The model under review builds one solid part; all positions refer to its coordinate system, in mm. A direction names the side the tool comes from. Round coordinates to 2 decimals unless told otherwise and drop trailing zeros. Loops run counter-clockwise (first coordinate to the right, second up) from the corner with the lowest first, then second, coordinate; pieces in that order, holes last. Notation, with made-up numbers: (67.5, -29.75) - (85.5, -29.75) arc R17 ccw to (85.5, -15.75) - close; hole circle Ø8 at (64, -31). An arc over 180 degrees is marked (long way). Answer as CSV lines item,"result".
from build123d import *

# Parameters (mm, degrees)
SKETCH1_W                                      = 104.000000026
SKETCH1_H                                      = 101.6
BOSS_EXTRUDE1_DEPTH                            = 10.16
SKETCH5_R                                      = 30.1625
BOSS_EXTRUDE2_DEPTH                            = 2.54
CBORE_FOR_6_SOCKET_HEAD_CAP_SCREW1_D           = 3.7973
CBORE_FOR_6_SOCKET_HEAD_CAP_SCREW1_CBORE_D     = 7.14502
CBORE_FOR_6_SOCKET_HEAD_CAP_SCREW1_CBORE_DEPTH = 3.5052
F_3_8_16_TAPPED_HOLE1_D                        = 7.9375
CBORE_FOR_M8_SBHCS1_D                          = 8.4
CBORE_FOR_M8_SBHCS1_CBORE_D                    = 14
CBORE_FOR_M8_SBHCS1_CBORE_DEPTH                = 4.4
CHAMFER1_SIZE                                  = 0.254
CHAMFER1_SIZE2                                 = 0.439940905
CHAMFER1_PART_2_SIZE                           = 0.254
CHAMFER1_PART_2_SIZE2                          = 0.439940905
CHAMFER2_SIZE                                  = 0.508


with BuildPart() as part:
    # Sketch1 → Boss-Extrude1 (new body)
    with BuildSketch(Plane(origin=(0, 0, 0), x_dir=(1, 0, 0), z_dir=(0, 1, 0))):
        with Locations((-52.000000013, 50.8)):
            Rectangle(SKETCH1_W, SKETCH1_H)
    extrude(amount=BOSS_EXTRUDE1_DEPTH)

    # Sketch5 → Boss-Extrude2 (add)
    with BuildSketch(Plane(origin=(0, 10.16, 0), x_dir=(1, 0, 0), z_dir=(0, 1, 0))):
        with Locations((-52.000000013, 62.5094)):
            Circle(SKETCH5_R)
    extrude(amount=BOSS_EXTRUDE2_DEPTH)

    # CBORE for #6 Socket Head Cap Screw1 (through all)
    with Locations(Plane(origin=(0, 10.16, 0), x_dir=(1, 0, 0), z_dir=(0, 1, 0))):
        with Locations((-44.380000013, 17.78), (-59.620000013, 17.78)):
            CounterBoreHole(CBORE_FOR_6_SOCKET_HEAD_CAP_SCREW1_D / 2, CBORE_FOR_6_SOCKET_HEAD_CAP_SCREW1_CBORE_D / 2, CBORE_FOR_6_SOCKET_HEAD_CAP_SCREW1_CBORE_DEPTH)

    # 3/8-16 Tapped Hole1 (through all)
    with Locations(Plane(origin=(0, 12.7, 0), x_dir=(1, 0, 0), z_dir=(0, 1, 0))):
        with Locations((-52.000000013, 62.5094)):
            Hole(F_3_8_16_TAPPED_HOLE1_D / 2)

    # CBORE for M8 SBHCS1 (through all)
    with Locations(Plane(origin=(0, 10.16, 0), x_dir=(1, 0, 0), z_dir=(0, 1, 0))):
        with Locations((-8.999999961, 92.6), (-8.999999961, 74.6), (-8.999999961, 27), (-8.999999961, 9), (-95.000000013, 9), (-95.000000013, 27), (-95.000000013, 74.6), (-95.000000013, 92.6)):
            CounterBoreHole(CBORE_FOR_M8_SBHCS1_D / 2, CBORE_FOR_M8_SBHCS1_CBORE_D / 2, CBORE_FOR_M8_SBHCS1_CBORE_DEPTH)

    # Chamfer1
    chamfer1_edges = [part.edges().sort_by_distance(p)[0] for p in [
        (0, 10.16, -50.8),
    ]]
    chamfer1_side = [part.faces().sort_by_distance(p)[0] for p in [
        (0, 5.08, -50.8),
    ]]
    chamfer(chamfer1_edges, length=CHAMFER1_SIZE, length2=CHAMFER1_SIZE2, reference=chamfer1_side[0])

    # Chamfer1 part 2
    chamfer1_part_2_edges = [part.edges().sort_by_distance(p)[0] for p in [
        (-104.000000026, 10.16, -50.8),
    ]]
    chamfer1_part_2_side = [part.faces().sort_by_distance(p)[0] for p in [
        (-104.000000026, 5.08, -50.8),
    ]]
    chamfer(chamfer1_part_2_edges, length=CHAMFER1_PART_2_SIZE, length2=CHAMFER1_PART_2_SIZE2, reference=chamfer1_part_2_side[0])

    # Chamfer2
    chamfer2_edges = [part.edges().sort_by_distance(p)[0] for p in [
        (0, 4.953, 0),
        (-104.000000026, 4.953, 0),
        (-104.000000026, 4.953, -101.6),
        (0, 4.953, -101.6),
    ]]
    chamfer(chamfer2_edges, length=CHAMFER2_SIZE)


solid = part.part
1. Clearance check with flat-ended pins moving along their axes: pin 1 (11 mm diameter, centred on x = -94.5, z = -91, fed in from +Y); pin 2 (7 mm diameter, centred on x = -11, z = -75, fed in from +Y). State where each tip first meets the part, or that it passes through.
Numbers:
pin 1,"stops at y = 10.16"
pin 2,"stops at y = 5.76"
2. Take a section at C-C (y = 1.25). State how many separate pieces and enclosed holes the cut face has, plus the area to 3 significant figures.
Numbers:
separate pieces,"1"
enclosed holes,"11"
area,"10,100 mm²"
3. Tool access review of faces 1 (the face through (-94.453, 2.84, -96.764)), 2 (the face through (-96.517, 7.991, -67.766)): name each direction out of +Z, -Z, +X, -X, +Y, -Y from which nothing blocks a thin tool from reaching the whole face with its end or side.
Numbers:
face 1,"+Y, -Y"
face 2,"+Y"
4. Take a section at D-D (z = -56.5). State the section outline as (x, y) points, plus the area to 3 significant figures.
Numbers:
outline,"(-104, 0) - (0, 0) - (0, 9.91) - (-0.44, 10.16) - (-22.44, 10.16) - (-22.44, 12.7) - (-81.56, 12.7) - (-81.56, 10.16) - (-103.56, 10.16) - (-104, 9.91) - close"
area,"1,210 mm²"
5. Take a section at B-B (x = -52). State the section outline as (y, z) points, plus the area to 3 significant figures.
Numbers:
outline,"(0, -101.6) - (10.16, -101.6) - (10.16, -92.67) - (12.7, -92.67) - (12.7, -66.48) - (0, -66.48) - close; (0, -58.54) - (12.7, -58.54) - (12.7, -32.35) - (10.16, -32.35) - (10.16, 0) - (0, 0) - close"
area,"1,080 mm²"
6. Take a section at A-A (z = -27). State the section outline as (x, y) points, plus the area to 3 significant figures.
Numbers:
outline,"(-104, 0) - (-99.2, 0) - (-99.2, 5.76) - (-102, 5.76) - (-102, 10.16) - (-103.56, 10.16) - (-104, 9.91) - close; (-90.8, 0) - (-13.2, 0) - (-13.2, 5.76) - (-16, 5.76) - (-16, 10.16) - (-88, 10.16) - (-88, 5.76) - (-90.8, 5.76) - close; (-4.8, 0) - (0, 0) - (0, 9.91) - (-0.44, 10.16) - (-2, 10.16) - (-2, 5.76) - (-4.8, 5.76) - close"
area,"837 mm²"
7. Wall thickness on probe 1 along Z at (x, y) = (-95, 3.45); probe 2 along Z at (x, y) = (-9, 8.35); probe 3 along X at (y, z) = (8.65, -74.6): over which ranges is each line inside the solid? List them lowest first.
Numbers:
probe 1,"z = -101.6 to -96.8, -88.4 to -78.8, -70.4 to -31.2, -22.8 to -13.2, -4.8 to 0"
probe 2,"z = -101.6 to -99.6, -85.6 to -81.6, -67.6 to -34, -20 to -16, -2 to 0"
probe 3,"x = -104 to -102, -88 to -16, -2 to 0"
8. Draft analysis for pull direction X (two halves, no side actions). For faces 3 (the face through (-8.453, 2.84, -96.764)), 4 (the face through (-53, 0, -52)), 5 (the face through (-104, 5, -50)), state which applies: +X half, -X half, draft (parallel to the pull), parting line (faces both ways), or undercut.
Numbers:
face 3,"undercut"
face 4,"draft"
face 5,"-X half"
